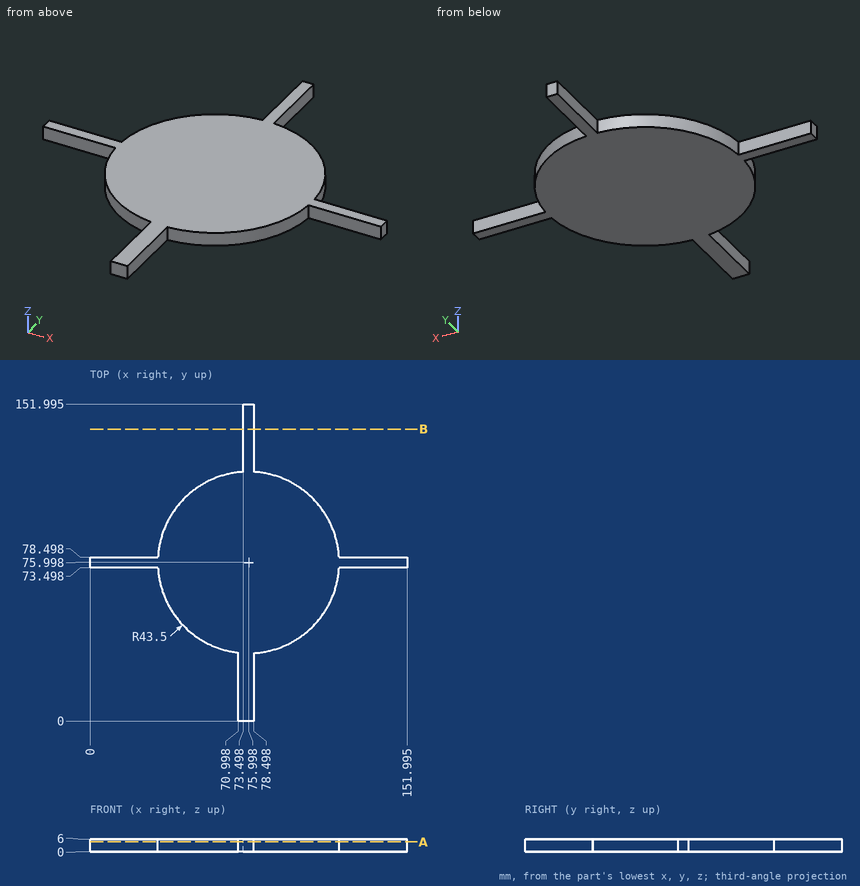
Input: dimensioned drawing with shaded views. Units: mm. Origin: part minimum x, y, z. Round coordinates to 2 decimals unless told otherwise and drop trailing zeros. Loops run counter-clockwise (first coordinate to the right, second up) from the corner with the lowest first, then second, coordinate; pieces in that order, holes last. Notation, with made-up numbers: M 3.25,37 L 21.25,37 A12 cw 21.25,48 Z; hole C 9.25,37 d2. An arc over 180 degrees is marked long. One line per question, with ' | ' between items.
(1) Contact query for flat-ended pins moving along their axis: P1, Ø8, axis at x = 105.5, y = 101.5, coming from the -Z side; P2, Ø3, axis at y = 131.5, z = 4, coming from the +X side; P3, Ø3, axis at x = 139, z = 4, coming from the -Y side; P4, Ø1.8, axis at y = 13.5, z = 1.5, coming from the -X side. Output: stop coordinate, or through.
Check result:
P1: stops at z = 0 | P2: stops at x = 78.5 | P3: stops at y = 73.5 | P4: stops at x = 71
(2) Cut plane A-A on z = 4.6. Return the cut outline in (x, y) (1 decimal).
Check result:
outline: M 0,73.5 L 32.6,73.5 A43.5 ccw 71,32.8 L 71,0 L 78.5,0 L 78.5,32.6 A43.5 ccw 119.4,73.5 L 152,73.5 L 152,78.5 L 119.4,78.5 A43.5 ccw 78.5,119.4 L 78.5,152 L 73.5,152 L 73.5,119.4 A43.5 ccw 32.6,78.5 L 0,78.5 Z
(3) Material intervals for line 1 along Y through (x, z) = (16, 0.55); line 2 along Y through (x, z) = (116, 1.4) (1 decimal); line 3 along X through (y, z) = (45, 4.2) (1 decimal), sorted ascending. Write a range as from..to.
Check result:
line 1: y = 73.5..78.5 | line 2: y = 58.9..93.1 | line 3: x = 45.5..106.5
(4) Cut plane B-B on y = 140. Return the cut outline in (x, z).
Check result:
outline: M 73.5,0 L 78.5,0 L 78.5,6 L 73.5,6 Z
